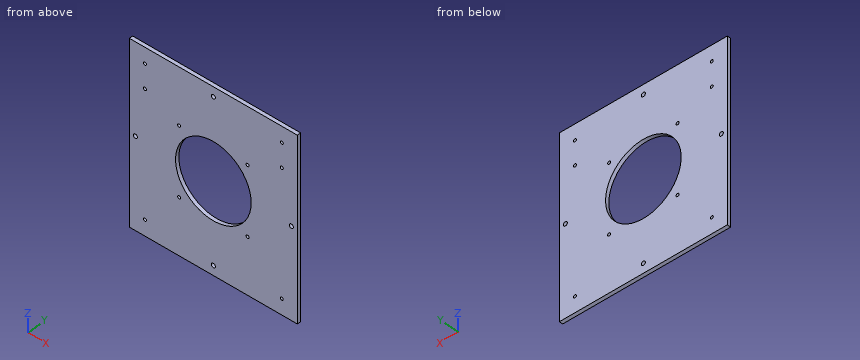
```python
from build123d import *

# Parameters (mm, degrees)
SKETCH_1_W           = 140
SKETCH_1_H           = 3
EXTRUDE_1_DEPTH      = 150
CUT_EXTRUDE_1_REACH  = 5
SKETCH_2_R           = 31.5
HOLE_WIZARD_M3_1_D   = 2.5
HOLE_WIZARD_M3_1_2_D = 3.4
HOLE_WIZARD_M3_2_D   = 2.5


with BuildPart() as part:
    # 草图1 → 拉伸-薄壁1 (new body)
    with BuildSketch(Plane.XY):
        with Locations((82, 225.557982809)):
            Rectangle(SKETCH_1_W, SKETCH_1_H)
    extrude(amount=EXTRUDE_1_DEPTH)

    # 草图2 → 切除-拉伸1 (cut, up to next)
    with BuildSketch(Plane.XZ.offset(-224.057982809), mode=Mode.PRIVATE) as cut_extrude_1_sk1:
        with Locations((82, 75)):
            Circle(SKETCH_2_R)
    cut_extrude_1_tool1 = extrude(cut_extrude_1_sk1.sketch, amount=-CUT_EXTRUDE_1_REACH, mode=Mode.PRIVATE) & part.part
    add(cut_extrude_1_tool1.solids().sort_by_distance((82, 224.057983, 75))[0], mode=Mode.SUBTRACT)

    # Hole Wizard M3 _1 (through all)
    with Locations(Plane(origin=(0, 224.057982809, 0), x_dir=(-1, 0, 0), z_dir=(0, -1, 0))):
        with Locations((-53.5, -103.5), (-53.5, -46.5), (-110.5, -46.5), (-110.5, -103.5)):
            Hole(HOLE_WIZARD_M3_1_D / 2)

    # Hole Wizard M3 _1 2 (through all)
    with Locations(Plane(origin=(0, 224.057982809, 0), x_dir=(-1, 0, 0), z_dir=(0, -1, 0))):
        with Locations((-82, -142), (-147, -75), (-82, -8), (-17, -75)):
            Hole(HOLE_WIZARD_M3_1_2_D / 2)

    # M3 螺纹孔的螺纹孔钻头2 (through all)
    with Locations(Plane(origin=(0, 224.057982809, 0), x_dir=(-1, 0, 0), z_dir=(0, -1, 0))):
        with Locations((-139, -137), (-139, -117), (-139, -13), (-25, -137), (-25, -117), (-25, -13)):
            Hole(HOLE_WIZARD_M3_2_D / 2)


solid = part.part
```
Can you work these out from the model? Positions are in its coordinate system, mm. Round coordinates to 2 decimals unless told otherwise and drop trailing zeros. Loops run counter-clockwise (first coordinate to the right, second up) from the corner with the lowest first, then second, coordinate; pieces in that order, holes last. Notation, with made-up numbers: (-2.5, 63) -> (27.5, 63) arc R21 ccw to (27.5, 91) -> close; hole circle Ø3 at (-28.75, -10.5). An arc over 180 degrees is marked (long way). One line per item, written item: value. Start each with the question number.
1. If we section it at A-A, the plane z = 75: Write out the boundary of the cut face in (x, y), then the cut area to 3 significant figures.
2. If I drill on probe 1 along X at (y, z) = (225.8, 117); probe 2 along Z at (x, y) = (25, 225.25); probe 3 along Z at (x, y) = (82, 226.4), over which ranges is the centre line in solid material (lowest first)?
3. If we section it at C-C, the plane z = 8: Write out the boundary of the cut face in (x, y).
4. If we section it at B-B, the plane x = 147: Write out the boundary of the cut face in (y, z), then the cut area to 3 significant figures.
5. If we section it at D-D, the plane y = 226.3: Give the number of separate pieces and of enclosed holes in the cut face, then the cut area to 3 significant figures.
6. For pin 1 (1.5 mm diameter, centred on x = 139, z = 117, fed in from -Y), with a flat end and sliding along its axis, tell me the tip position at first contact or that it passes through.
Calculated:
1. outline: (12, 224.06) -> (15.3, 224.06) -> (15.3, 227.06) -> (12, 227.06) -> close; (18.7, 224.06) -> (50.5, 224.06) -> (50.5, 227.06) -> (18.7, 227.06) -> close; (113.5, 224.06) -> (145.3, 224.06) -> (145.3, 227.06) -> (113.5, 227.06) -> close; (148.7, 224.06) -> (152, 224.06) -> (152, 227.06) -> (148.7, 227.06) -> close
1. area: 211 mm²
2. probe 1: x = 12 to 23.75, 26.25 to 137.75, 140.25 to 152
2. probe 2: z = 0 to 11.75, 14.25 to 115.75, 118.25 to 135.75, 138.25 to 150
2. probe 3: z = 0 to 6.3, 9.7 to 43.5, 106.5 to 140.3, 143.7 to 150
3. outline: (12, 224.06) -> (80.3, 224.06) -> (80.3, 227.06) -> (12, 227.06) -> close; (83.7, 224.06) -> (152, 224.06) -> (152, 227.06) -> (83.7, 227.06) -> close
4. outline: (224.06, 0) -> (227.06, 0) -> (227.06, 73.3) -> (224.06, 73.3) -> close; (224.06, 76.7) -> (227.06, 76.7) -> (227.06, 150) -> (224.06, 150) -> close
4. area: 440 mm²
5. separate pieces: 1
5. enclosed holes: 15
5. area: 17,800 mm²
6. pin 1: passes through
